Verification items for this drawing (mm, ordinates from the low corner). A direction names the side the tool comes from. Round coordinates to 2 decimals unless told otherwise and drop trailing zeros. Write each loop counter-clockwise with the first axis right and the second up, starting at its lowest first coordinate (ties: lowest second). Pieces come first, ordered by that corner, then holes.
Item 1: Cross-section at C-C (y = 1). Enter the section's corners in (x, z), then the cut area to 3 significant figures.
Item 2: Depth check by flat-ended pin: P1, Ø1.5, axis at x = 5, z = 28.5, coming from the -Y side (1 decimal); P2, Ø2, axis at x = 1, z = 8.5, coming from the -Y side. Enter the tip coordinate at first touch or a pass-through.
Item 3: Access from +Z, -Z, +X, -X, +Y, -Y to the whole of each face (thin tool, end or side, straight path). Record for the marked faces 1 and 2.
Item 4: Scan lines: probe 1 along Z at (x, y) = (0.7, 3); probe 2 along Y at (x, z) = (3.65, 2.5) (1 decimal); probe 3 along Y at (x, z) = (2.05, 5) (1 decimal). Record each from-to range of solid material in increasing order.
Item 5: Cross-section at B-B (x = 0.45). Enter the section's corners in (y, z).
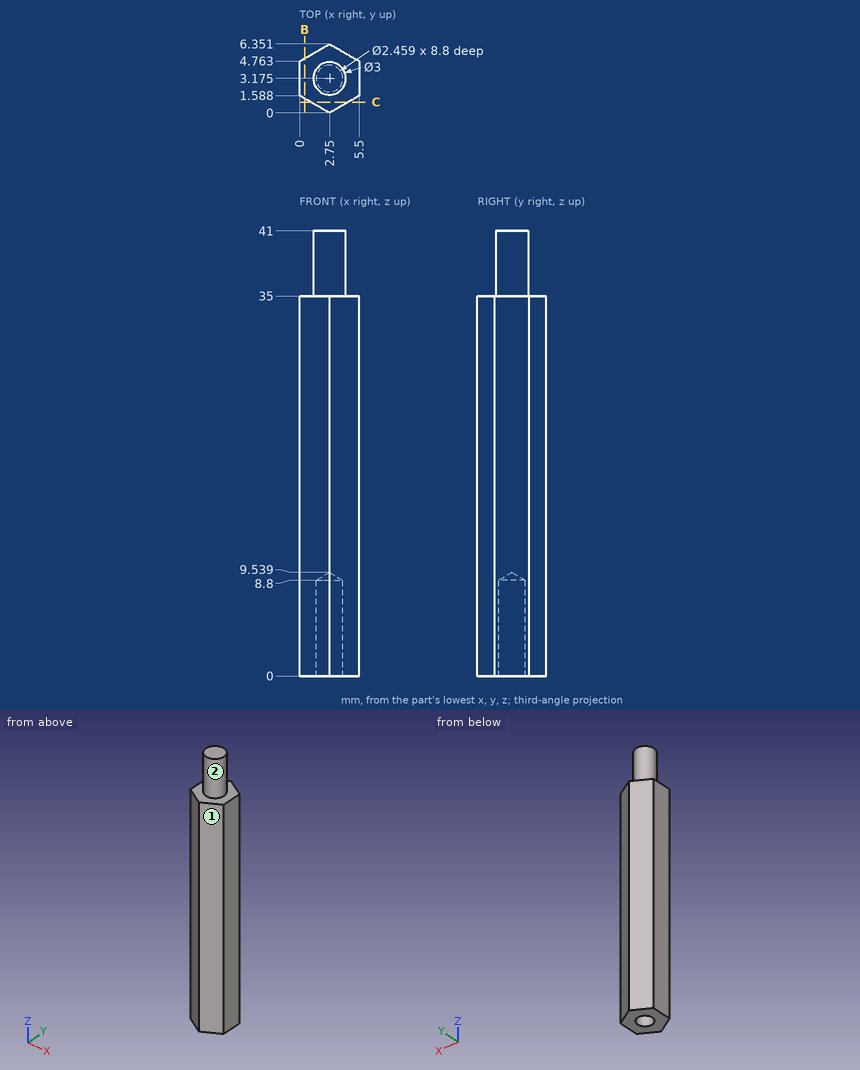
Resolved:
1. outline: (1.02, 0) - (4.48, 0) - (4.48, 35) - (1.02, 35) - close
1. area: 121 mm2
2. P1: stops at y = 0.9
2. P2: stops at y = 0.43
3. face 1: +Z, -Z, +X, -Y
3. face 2: +Z
4. probe 1: z = 0 to 35
4. probe 2: y = 0.5 to 2.3, 4 to 5.8
4. probe 3: y = 0.4 to 2.2, 4.2 to 5.9
5. outline: (1.33, 0) - (5.02, 0) - (5.02, 35) - (1.33, 35) - close
